Source: CAD feature listing. Evaluate the final solid. Frame: model axes, mm. A direction names the side the tool comes from. Round coordinates to 2 decimals unless told otherwise and drop trailing zeros. Order: outer loops, then holes, each group sorted by start corner. A loop starts at its lowest first (then second) coordinate and runs counter-clockwise, first axis right, second up. Notation, with made-up numbers: (73.25, 46.5) -> (91.25, 46.5) arc R20 ccw to (91.25, 84.5) -> close; hole circle Ø2 at (82.5, -39). An arc over 180 degrees is marked (long way). Answer as CSV lines item,"result".
from build123d import *

# Parameters (mm, degrees)
EXTRUDE_2_DEPTH = 29.8
FILLET_3_R      = 2.5


with BuildPart() as part:
    # Эскиз1 → Бобышка-Вытянуть2 (new body)
    with BuildSketch(Plane.XY):
        with BuildLine():
            Line((0, 0), (79.5, 0))
            Line((79.5, 0), (79.5, 5))
            Line((79.5, 5), (69, 5))
            Line((69, 5), (69, 10.4))
            Line((69, 10.4), (77, 10.4))
            ThreePointArc((77, 10.4), (78.767766953, 11.132233047), (79.5, 12.9))
            Line((79.5, 12.9), (79.5, 30.395890056))
            ThreePointArc((79.5, 30.395890056), (76.571067812, 37.466957868), (69.5, 40.395890056))
            Line((69.5, 40.395890056), (10, 40.395890056))
            ThreePointArc((10, 40.395890056), (2.928932188, 37.466957868), (0, 30.395890056))
            Line((0, 30.395890056), (0, 12.9))
            ThreePointArc((0, 12.9), (0.732233047, 11.132233047), (2.5, 10.4))
            Line((2.5, 10.4), (10.5, 10.4))
            Line((10.5, 10.4), (10.5, 5))
            Line((10.5, 5), (0, 5))
            Line((0, 5), (0, 0))
        make_face()
        with BuildLine():
            Line((10, 35.395890056), (69.5, 35.395890056))
            ThreePointArc((69.5, 35.395890056), (73.035533906, 33.931423962), (74.5, 30.395890056))
            Line((74.5, 30.395890056), (74.5, 20.4))
            ThreePointArc((74.5, 20.4), (73.035533906, 16.864466094), (69.5, 15.4))
            Line((69.5, 15.4), (10, 15.4))
            ThreePointArc((10, 15.4), (6.464466094, 16.864466094), (5, 20.4))
            Line((5, 20.4), (5, 30.395890056))
            ThreePointArc((5, 30.395890056), (6.464466094, 33.931423962), (10, 35.395890056))
        make_face(mode=Mode.SUBTRACT)
    extrude(amount=EXTRUDE_2_DEPTH)

    # Скругление3
    fillet_3_edges = [part.edges().sort_by_distance(p)[0] for p in [
        (6.5, 10.4, 0),
        (0.732233047, 11.132233047, 0),
        (0, 21.647945028, 0),
        (2.928932188, 37.466957868, 0),
        (39.75, 40.395890056, 0),
        (76.571067812, 37.466957868, 0),
        (79.5, 21.647945028, 0),
        (78.767766953, 11.132233047, 0),
        (73, 10.4, 0),
        (73, 10.4, 29.8),
        (78.767766953, 11.132233047, 29.8),
        (79.5, 21.647945028, 29.8),
        (76.571067812, 37.466957868, 29.8),
        (39.75, 40.395890056, 29.8),
        (2.928932188, 37.466957868, 29.8),
        (73.035533906, 33.931423962, 0),
        (39.75, 35.395890056, 0),
        (6.464466094, 33.931423962, 0),
        (5, 25.397945028, 0),
        (6.464466094, 16.864466094, 0),
        (39.75, 15.4, 0),
        (73.035533906, 16.864466094, 0),
        (74.5, 25.397945028, 0),
        (0, 21.647945028, 29.8),
        (73.035533906, 33.931423962, 29.8),
        (39.75, 35.395890056, 29.8),
        (6.464466094, 33.931423962, 29.8),
        (5, 25.397945028, 29.8),
        (6.464466094, 16.864466094, 29.8),
        (39.75, 15.4, 29.8),
        (73.035533906, 16.864466094, 29.8),
        (74.5, 25.397945028, 29.8),
        (0.732233047, 11.132233047, 29.8),
        (6.5, 10.4, 29.8),
    ]]
    fillet(fillet_3_edges, radius=FILLET_3_R - 0.0001)  # a hair under: the kernel refuses the full size


solid = part.part
1. Mould query, pull axis X, two halves, no side actions, for faces 5 (the flat face through (79.5, 2, 15)), 6 (the cylindrical face through (39.334, 14.687, 0.752)), 7 (the flat face through (5, 5, 15)). Classes: released by +X, released by -X, zero draft, split by the parting line, or undercut.
Results below:
face 5,"released by +X"
face 6,"undercut"
face 7,"zero draft"
2. Section query D-D on y = 9. Return loops of the section in (x, z), and give its area (3 significant figures).
Results below:
outline,"(10.5, 0) -> (69, 0) -> (69, 29.8) -> (10.5, 29.8) -> close"
area,"1,740 mm2"
3. Reachability of faces 1 (the flat face through (40, 15.4, 15)), 2 (the cylindrical face through (79, 22, 1)), 3 (the cylindrical face through (4.287, 25.468, 0.752)), 4 (the flat face through (6, 10.4, 15)) from +Z, -Z, +X, -X, +Y, -Y: full face, straight path, thin tool, end or side. Return the list, or none.
Results below:
face 1,"+Z, -Z"
face 2,"-Z, +X, +Y"
face 3,"-Z"
face 4,"+Z, -Z, -X"
4. Pin query (flat end, axial travel): pin 1 (5 mm diameter, centred on x = 74, z = 19.5, fed in from +Y); pin 2 (2.5 mm diameter, centred on y = 7, z = 12.5, fed in from -X); pin 3 (3 mm diameter, centred on x = 6, z = 13, fed in from +Y). Return the tip coordinate at first contact, or that it passes through.
Results below:
pin 1,"y = 40.19"
pin 2,"x = 10.5"
pin 3,"y = 40.08"
5. Section query B-B on z = 19.5. Return loops of the section in (x, y), and give its area (3 significant figures).
Results below:
outline,"(0, 0) -> (79.5, 0) -> (79.5, 5) -> (69, 5) -> (69, 10.4) -> (77, 10.4) arc R2.5 ccw to (79.5, 12.9) -> (79.5, 30.4) arc R10 ccw to (69.5, 40.4) -> (10, 40.4) arc R10 ccw to (0, 30.4) -> (0, 12.9) arc R2.5 ccw to (2.5, 10.4) -> (10.5, 10.4) -> (10.5, 5) -> (0, 5) -> close; hole (5, 20.4) arc R5 ccw to (10, 15.4) -> (69.5, 15.4) arc R5 ccw to (74.5, 20.4) -> (74.5, 30.4) arc R5 ccw to (69.5, 35.4) -> (10, 35.4) arc R5 ccw to (5, 30.4) -> close"
area,"1,680 mm2"
6. Line query: L1, parallel to X at y = 22.5, z = 10.75; L2, parallel to Y at x = 26, z = 24.75; L3, parallel to Y at x = 9, z = 17.5. Output: solid intervals per line, ascending. Write a range as [from, to].
Results below:
L1,"[0, 5], [74.5, 79.5]"
L2,"[0, 15.4], [35.4, 40.4]"
L3,"[0, 5], [10.4, 15.5], [35.29, 40.35]"
